Read the model definition and answer for the solid it produces. Units are mm, in the model's axes. Face numbers are marked on the shaded views. Coordinates: 2 decimals unless noted, no trailing zeros. Write each loop counter-clockwise with the first axis right and the second up, starting at its lowest first coordinate (ties: lowest second). Pieces come first, ordered by that corner, then holes.
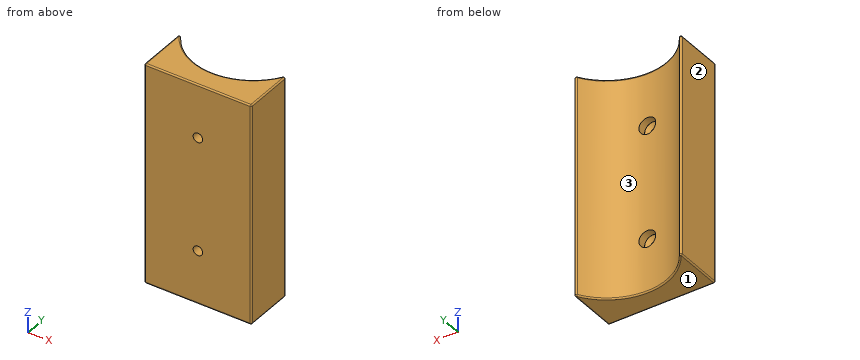
from build123d import *

# Parameters (mm, degrees)
BOSS_EXTRUDE1_DEPTH                                 = 83.82
FILLET1_R                                           = 0.508
CUT_EXTRUDE1_START                                  = 5.08
SKETCH5_R                                           = 3.175
CUT_EXTRUDE1_DEPTH                                  = 90.986026172
CSK_FOR_M3_COUNTERSUNK_FLAT_HEAD_SCREW1_D           = 3.6
CSK_FOR_M3_COUNTERSUNK_FLAT_HEAD_SCREW1_DEPTH       = 419.354
CSK_FOR_M3_COUNTERSUNK_FLAT_HEAD_SCREW1_CSINK_D     = 6.3
CSK_FOR_M3_COUNTERSUNK_FLAT_HEAD_SCREW1_CSINK_ANGLE = 90
CSK_FOR_M3_COUNTERSUNK_FLAT_HEAD_SCREW1_TIP         = 1.081549114
FILLET2_R                                           = 0.508


with BuildPart() as part:
    # Sketch2 → Boss-Extrude1 (new body)
    with BuildSketch(Plane.XY):
        with BuildLine():
            Line((0, 0), (40.64, 0))
            Line((40.64, 0), (40.64, 20.388311711))
            ThreePointArc((40.64, 20.388311711), (20.32, 8.001), (0, 20.388311711))
            Line((0, 20.388311711), (0, 0))
        make_face()
    extrude(amount=BOSS_EXTRUDE1_DEPTH)

    # Fillet1
    fillet1_edges = [part.edges().sort_by_distance(p)[0] for p in [
        (0, 20.388311711, 41.91),
        (40.64, 20.388311711, 41.91),
    ]]
    fillet(fillet1_edges, radius=FILLET1_R)

    # Sketch5 → Cut-Extrude1 (cut, through all)
    with BuildSketch(Plane(origin=(0, 0, 0), x_dir=(1, 0, 0), z_dir=(0, 1, 0)).offset(CUT_EXTRUDE1_START)):
        with Locations(Location((20.32, -20.32, 0), (0, 0, 90))):
            Circle(SKETCH5_R)
        with Locations(Location((20.32, -63.5, 0), (0, 0, 90))):
            Circle(SKETCH5_R)
    extrude(amount=CUT_EXTRUDE1_DEPTH, mode=Mode.SUBTRACT)

    # CSK for M3 Countersunk Flat Head Screw1
    with Locations(Plane(origin=(0, 5.08, 0), x_dir=(1, 0, 0), z_dir=(0, 1, 0))):
        with Locations((20.32, -20.32), (20.32, -63.5)):
            CounterSinkHole(CSK_FOR_M3_COUNTERSUNK_FLAT_HEAD_SCREW1_D / 2, CSK_FOR_M3_COUNTERSUNK_FLAT_HEAD_SCREW1_CSINK_D / 2, depth=CSK_FOR_M3_COUNTERSUNK_FLAT_HEAD_SCREW1_DEPTH, counter_sink_angle=CSK_FOR_M3_COUNTERSUNK_FLAT_HEAD_SCREW1_CSINK_ANGLE)
            with Locations((0, 0, -(CSK_FOR_M3_COUNTERSUNK_FLAT_HEAD_SCREW1_DEPTH + CSK_FOR_M3_COUNTERSUNK_FLAT_HEAD_SCREW1_TIP / 2))):  # 118° drill point
                Cone(0, CSK_FOR_M3_COUNTERSUNK_FLAT_HEAD_SCREW1_D / 2, CSK_FOR_M3_COUNTERSUNK_FLAT_HEAD_SCREW1_TIP, mode=Mode.SUBTRACT)

    # Fillet2
    fillet2_edges = [part.edges().sort_by_distance(p)[0] for p in [
        (40.64, 9.234774054, 83.82),
        (20.32, 8.001, 0),
        (20.32, 8.001, 83.82),
        (0, 9.234774054, 0),
        (0.36787397, 18.957839717, 0),
        (40.27212603, 18.957839717, 0),
        (0, 9.234774054, 83.82),
        (0.36787397, 18.957839717, 83.82),
        (40.27212603, 18.957839717, 83.82),
        (40.64, 9.234774054, 0),
        (20.32, 0, 0),
        (40.64, 0, 41.91),
        (0, 0, 41.91),
        (20.32, 0, 83.82),
    ]]
    fillet(fillet2_edges, radius=FILLET2_R)


solid = part.part
Item 1: The part is cut by section B-B (z = 20.32). Give the vertices of the cut face in (x, y) (3 decimals), and give its area (3 significant figures).
Item 2: The part is cut by section A-A (x = 20.32). Give the vertices of the cut face in (y, z) (3 decimals), and give its area (3 significant figures).
Item 3: Given pin 1 (5 mm diameter, centred on x = 19, z = 19, fed in from +Y); pin 2 (3 mm diameter, centred on x = 21.5, z = 64, fed in from +Y); pin 3 (3 mm diameter, centred on x = 25.5, y = 10.5, fed in from -Z), each flat-ended and moving along its own axis, determine where each tip first touches the part or whether it passes through.
Item 4: The part is cut by section C-C (z = 78). Give the vertices of the cut face in (x, y), and give its area (3 significant figures).
Item 5: Find the intervals of material crossed by probe 1 along Z at (x, y) = (20.32, 6.1) (3 decimals); probe 2 along Z at (x, y) = (20.32, 2.75); probe 3 along X at (y, z) = (5.8, 63.5) (3 decimals), in increasing order.
Item 6: Determine the mould class of the marked faces 1, 2 and 3 for opening direction X: +X half, -X half, draft (parallel to the pull), parting line (faces both ways), or undercut.
Answer:
1. outline: (0, 0.508) arc R0.508 ccw to (0.508, 0) - (18.52, 0) - (18.52, 3.73) - (17.17, 5.08) - (17.145, 5.08) - (17.145, 8.223) arc R22.86 cw to (0.939, 18.739) arc R0.508 ccw to (0, 18.47) - close; (22.12, 0) - (40.132, 0) arc R0.508 ccw to (40.64, 0.508) - (40.64, 18.47) arc R0.508 ccw to (39.701, 18.739) arc R22.86 cw to (23.495, 8.223) - (23.495, 5.08) - (23.47, 5.08) - (22.12, 3.73) - close
1. area: 429 mm2
2. outline: (0, 0.508) arc R0.508 ccw to (0.508, 0) - (7.493, 0) arc R0.508 ccw to (8.001, 0.508) - (8.001, 17.145) - (5.08, 17.145) - (5.08, 17.17) - (3.73, 18.52) - (0, 18.52) - close; (0, 22.12) - (3.73, 22.12) - (5.08, 23.47) - (5.08, 23.495) - (8.001, 23.495) - (8.001, 60.325) - (5.08, 60.325) - (5.08, 60.35) - (3.73, 61.7) - (0, 61.7) - close; (0, 65.3) - (3.73, 65.3) - (5.08, 66.65) - (5.08, 66.675) - (8.001, 66.675) - (8.001, 83.312) arc R0.508 ccw to (7.493, 83.82) - (0.508, 83.82) arc R0.508 ccw to (0, 83.312) - close
2. area: 593 mm2
3. pin 1: stops at y = 8.32
3. pin 2: stops at y = 4.71
3. pin 3: passes through
4. outline: (0, 0.51) arc R0.51 ccw to (0.51, 0) - (40.13, 0) arc R0.51 ccw to (40.64, 0.51) - (40.64, 18.47) arc R0.51 ccw to (39.7, 18.74) arc R22.86 cw to (0.94, 18.74) arc R0.51 ccw to (0, 18.47) - close
4. area: 468 mm2
5. probe 1: z = 0 to 17.145, 23.495 to 60.325, 66.675 to 83.82
5. probe 2: z = 0 to 18.52, 22.12 to 61.7, 65.3 to 83.82
5. probe 3: x = 0 to 17.145, 23.495 to 40.64
6. face 1: draft
6. face 2: -X half
6. face 3: undercut
